Verification items for the finished model (mm, model axes). Face numbers are marked on the shaded views. Round coordinates to 2 decimals unless told otherwise and drop trailing zeros. Write each loop counter-clockwise with the first axis right and the second up, starting at its lowest first coordinate (ties: lowest second). Pieces come first, ordered by that corner, then holes. Notation, with made-up numbers: (48, 55.25) -> (102, 55.25) arc R34 ccw to (102, 88.25) -> close; hole circle Ø1 at (57.5, 56). An arc over 180 degrees is marked (long way). Answer as a JSON object with one key per item and string values. Group by question number.
(1) Sectioned sample at C-C on y = 1.75. Record the cut outline in (x, z) (3 decimals).
(2) Sectioned sample at D-D on x = 26. Record the cut outline in (y, z), and give its area (3 significant figures).
(3) Sectioned sample at A-A on x = 0. Record the cut outline in (y, z) (3 decimals).
(4) Gauge pin test, flat ends, axial feed: pin 1 Ø2 at (y, z) = (1.5, -0.5) entering from -X; pin 2 Ø12 at (x, z) = (28, -4.5) entering from -Y; pin 3 Ø1.5 at (y, z) = (1, -40.5) entering from -X; pin 4 Ø1.5 at (y, z) = (1.5, -31.5) entering from +X. Record the tip position at first contact, or that the pin passes through.
(5) Scan lines: L1, parallel to Z at x = 0, y = 4.25 (3 decimals); L2, parallel to X at y = 3, z = -12.7; L3, parallel to Z at x = -25.4, y = 2.5. Record each from-to range of solid material in increasing order. Write a range as from..to.
(6) Sectioned sample at B-B on z = 0. Record the cut outline in (x, y) (3 decimals).
(7) Draft check along Z on the marked faces 1, 2 and 3. Enter one of: released by +Z, released by -Z, zero draft, split by the parting line, or undercut.
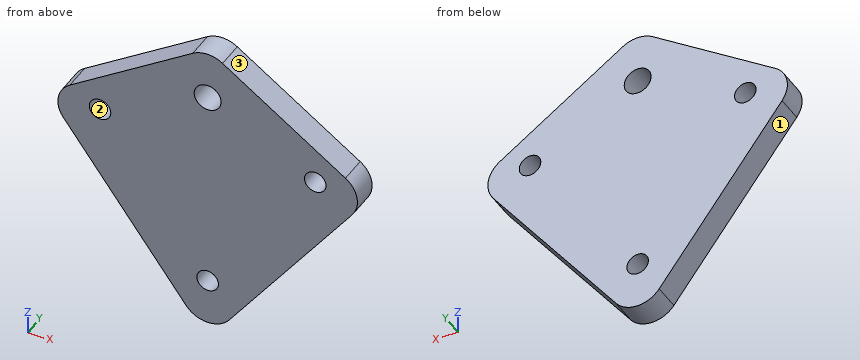
```python
from build123d import *

# Parameters (mm, degrees)
SKETCH2_R           = 3.175
SKETCH2_R_2         = 2.54
BOSS_EXTRUDE2_DEPTH = 6.35
FILLET3_R           = 6.35


with BuildPart() as part:
    # Sketch2 → Boss-Extrude2 (new body)
    with BuildSketch(Plane(origin=(0, 0, 0), x_dir=(1, 0, 0), z_dir=(0, 1, 0))):
        Polygon((0, 63.5), (-38.1, 12.7), (0, -12.7), (38.1, 12.7), align=None)
        Circle(SKETCH2_R, mode=Mode.SUBTRACT)
        with Locations((-25.4, 12.7)):
            Circle(SKETCH2_R_2, mode=Mode.SUBTRACT)
        with Locations((0, 48.26)):
            Circle(SKETCH2_R_2, mode=Mode.SUBTRACT)
        with Locations((25.4, 12.7)):
            Circle(SKETCH2_R_2, mode=Mode.SUBTRACT)
    extrude(amount=BOSS_EXTRUDE2_DEPTH)

    # Fillet3
    fillet3_edges = [part.edges().sort_by_distance(p)[0] for p in [
        (0, 3.175, 12.7),
        (-38.1, 3.175, -12.7),
        (0, 3.175, -63.5),
        (38.1, 3.175, -12.7),
    ]]
    fillet(fillet3_edges, radius=FILLET3_R)


solid = part.part
```
Computed values:
{
 "1": {"outline": "(-34.072, -18.07) -> (-5.08, -56.727) arc R6.35 ccw to (5.08, -56.727) -> (34.072, -18.07) arc R6.35 ccw to (32.515, -8.977) -> (3.522, 10.352) arc R6.35 ccw to (-3.522, 10.352) -> (-32.515, -8.977) arc R6.35 ccw to start; hole circle Ø5.08 at (-25.4, -12.7); hole circle Ø6.35 at (0, 0); hole circle Ø5.08 at (0, -48.26); hole circle Ø5.08 at (25.4, -12.7)"},
 "2": {"outline": "(0, -28.83) -> (6.35, -28.83) -> (6.35, -15.17) -> (0, -15.17) -> close; (0, -10.23) -> (6.35, -10.23) -> (6.35, -4.63) -> (0, -4.63) -> close", "area": "122 mm2"},
 "3": {"outline": "(0, -59.267) -> (6.35, -59.267) -> (6.35, -50.8) -> (0, -50.8) -> close; (0, -45.72) -> (6.35, -45.72) -> (6.35, -3.175) -> (0, -3.175) -> close; (0, 3.175) -> (6.35, 3.175) -> (6.35, 11.418) -> (0, 11.418) -> close"},
 "4": {"pin 1": "x = -21.3", "pin 2": "y = 0", "pin 3": "x = -17.81", "pin 4": "x = 24.56"},
 "5": {"L1": "-59.267..-50.8, -45.72..-3.175, 3.175..11.418", "L2": "-35.15..-27.94, -22.86..22.86, 27.94..35.15", "L3": "-29.63..-15.24, -10.16..-4.23"},
 "6": {"outline": "(-19.05, 0) -> (-3.175, 0) -> (-3.175, 6.35) -> (-19.05, 6.35) -> close; (3.175, 0) -> (19.05, 0) -> (19.05, 6.35) -> (3.175, 6.35) -> close"},
 "7": {"face 1": "released by -Z", "face 2": "undercut", "face 3": "released by +Z"}
}
